Geometry: final body of the model. Coordinates: model frame, mm. A direction names the side the tool comes from. Give positions to 0.01 mm unless a question says otherwise; leave off trailing zeros. Write each loop counter-clockwise with the first axis right and the second up, starting at its lowest first coordinate (ties: lowest second). Pieces come first, ordered by that corner, then holes. Notation, with made-up numbers: (54.25, 1) - (84.25, 1) arc R24 ccw to (84.25, 37) - close; hole circle Ø1 at (79, 28). An arc over 180 degrees is marked (long way). Return JSON: item names as keys, results as strings.
from build123d import *

# Parameters (mm, degrees)
SKETCH1_R           = 1.27
BOSS_EXTRUDE1_DEPTH = 2.286
SKETCH2_R           = 2.032
BOSS_EXTRUDE2_DEPTH = 1.016
SKETCH3_R           = 1.524
BOSS_EXTRUDE3_DEPTH = 0.889
SKETCH4_R           = 2.032
BOSS_EXTRUDE4_DEPTH = 2.159
SKETCH6_R           = 3.1115
BOSS_EXTRUDE5_DEPTH = 3.937
SKETCH7_R           = 2.032
BOSS_EXTRUDE6_DEPTH = 1.27
SKETCH8_R           = 1.524
BOSS_EXTRUDE7_DEPTH = 0.889
SKETCH9_R           = 2.032
BOSS_EXTRUDE8_DEPTH = 11.43
FILLET1_R           = 2.032


with BuildPart() as part:
    # Sketch1 → Boss-Extrude1 (new body)
    with BuildSketch(Plane.XY):
        Circle(SKETCH1_R)
    extrude(amount=BOSS_EXTRUDE1_DEPTH)

    # Sketch2 → Boss-Extrude2 (add)
    with BuildSketch(Plane.XY.offset(2.286)):
        Circle(SKETCH2_R)
    extrude(amount=BOSS_EXTRUDE2_DEPTH)

    # Sketch3 → Boss-Extrude3 (add)
    with BuildSketch(Plane.XY.offset(3.302)):
        Circle(SKETCH3_R)
    extrude(amount=BOSS_EXTRUDE3_DEPTH)

    # Sketch4 → Boss-Extrude4 (add)
    with BuildSketch(Plane.XY.offset(4.191)):
        Circle(SKETCH4_R)
    extrude(amount=BOSS_EXTRUDE4_DEPTH)

    # Sketch6 → Boss-Extrude5 (add)
    with BuildSketch(Plane.XY.offset(6.35)):
        Circle(SKETCH6_R)
    extrude(amount=BOSS_EXTRUDE5_DEPTH)

    # Sketch7 → Boss-Extrude6 (add)
    with BuildSketch(Plane.XY.offset(10.287)):
        Circle(SKETCH7_R)
    extrude(amount=BOSS_EXTRUDE6_DEPTH)

    # Sketch8 → Boss-Extrude7 (add)
    with BuildSketch(Plane.XY.offset(11.557)):
        Circle(SKETCH8_R)
    extrude(amount=BOSS_EXTRUDE7_DEPTH)

    # Sketch9 → Boss-Extrude8 (add)
    with BuildSketch(Plane.XY.offset(12.446)):
        Circle(SKETCH9_R)
    extrude(amount=BOSS_EXTRUDE8_DEPTH)

    # Fillet1
    fillet1_edges = [part.edges().sort_by_distance(p)[0] for p in [
        (-2.032, 0, 23.876),
    ]]
    fillet(fillet1_edges, radius=FILLET1_R)


solid = part.part
Q1. Pin query (flat end, axial travel): P1, Ø2, axis at x = 1.5, y = -1.5, coming from the -Z side; P2, Ø1.9, axis at x = -1.5, y = 0.5, coming from the +Z side; P3, Ø1.5, axis at x = -1.5, z = 10.5, coming from the -Y side. Return the tip coordinate at first contact, or that it passes through.
Answer key:
{"P1": "stops at z = 0", "P2": "stops at z = 23.78", "P3": "stops at y = -3.01"}
Q2. Set-up query: faces 1 (the cylindrical face through (-0.44, -1.984, 17.079)), 2 (the cylindrical face through (-0.2, 1.51, 3.74)), 3 (the cylindrical face through (-0.44, -1.984, 5.255)). Return all of +Z, -Z, +X, -X, +Y, -Y with unobstructed straight access to the full face (end or side cutting, diameter ignored); none if empty.
Answer key:
{"face 1": "+Z", "face 2": "none", "face 3": "-Z"}
Q3. Section query C-C, the plane z = 17. Return the cut outline in (x, y).
Answer key:
{"outline": "circle Ø4.06 at (0, 0)"}
Q4. Mould query, pull axis Z, two halves, no side actions, for faces 4 (the cylindrical face through (-0.67, -3.04, 8.29)), 5 (the cylindrical face through (-0.2, 1.51, 12)), 6 (the flat face through (0, 0, 0)). Classes: pulls with the +Z half, pulls with the -Z half, needs draft (parallel to the pull), parting line crosses it, or undercut.
Answer key:
{"face 4": "needs draft", "face 5": "undercut", "face 6": "pulls with the -Z half"}
Q5. Material intervals for probe 1 along Z at (x, y) = (-2.25, 0.75); probe 2 along Z at (x, y) = (1.75, -0.5); probe 3 along X at (y, z) = (1.5, 7), sorted ascending. Write a range as [from, to].
Answer key:
{"probe 1": "z = [6.35, 10.29]", "probe 2": "z = [2.29, 3.3], [4.19, 11.56], [12.45, 22.75]", "probe 3": "x = [-2.73, 2.73]"}
Q6. Section query D-D, the plane x = 2.75. Return the cut outline in (y, z).
Answer key:
{"outline": "(-1.46, 6.35) - (1.46, 6.35) - (1.46, 10.29) - (-1.46, 10.29) - close"}
